Can you work these out from the model? Positions are in its coordinate system, mm. Face numbers are marked on the shaded views. A direction names the side the tool comes from. Round coordinates to 2 decimals unless told otherwise and drop trailing zeros. Write each loop counter-clockwise with the first axis right and the second up, starting at its lowest first coordinate (ties: lowest second). Pieces come first, ordered by that corner, then holes. Notation, with made-up numbers: (3, 6) -> (52, 6) arc R15 cw to (52, 19) -> close; hole circle Ø9 at (68, 46.25). An arc over 180 degrees is marked (long way). Use CSV: the item, a comma, the result in double quotes.
```python
from build123d import *

# Parameters (mm, degrees)
SKETCH1_R                            = 20.334999999999997
SKETCH1_R_2                          = 13.334999999999999
BOSS_EXTRUDE1_DEPTH                  = 12
BOSS_EXTRUDE2_DEPTH                  = 10
BOSS_EXTRUDE2_DIRECTION_2_REACH      = 49.027
BOSS_EXTRUDE2_DIRECTION_2_END_RADIUS = 13.334999999999999
CUT_EXTRUDE1_REACH                   = 62.473
CUT_EXTRUDE1_END_RADIUS              = 20.334999999999997
BOSS_EXTRUDE3_DEPTH                  = 11


with BuildPart() as part:
    # Sketch1 → Boss-Extrude1 (new body)
    with BuildSketch(Plane(origin=(0, 0, 0), x_dir=(1, 0, 0), z_dir=(0, 1, 0))):
        with Locations(Location((0, 0, 0), (0, 0, 270))):
            Circle(SKETCH1_R)
        with Locations(Location((0, 0, 0), (0, 0, 270))):
            Circle(SKETCH1_R_2, mode=Mode.SUBTRACT)
    extrude(amount=BOSS_EXTRUDE1_DEPTH)

    # Sketch2 → Boss-Extrude2 (add)
    with BuildSketch(Plane.XY.offset(20.334999999999997)):
        Polygon((-8, 26.000000000000004), (-7.9999999999999964, 0), (8.000000000000004, 0), (8, 26.000000000000004), align=None)
        Polygon((-5.000000000000001, 23.000000000000004), (5, 23.000000000000004), (4.999999999999998, 3), (-4.999999999999998, 3), align=None, mode=Mode.SUBTRACT)
    extrude(amount=BOSS_EXTRUDE2_DEPTH)

    # Boss-Extrude2 direction 2: up to this cylinder (the profile starts outside it)
    boss_extrude2_direction_2_end = Plane(origin=(0, 13, 0), z_dir=(0, -1, 0)) * Cylinder(BOSS_EXTRUDE2_DIRECTION_2_END_RADIUS, 125.724, mode=Mode.PRIVATE)
    # Sketch2 → Boss-Extrude2 direction 2 (add, up to the surface)
    with BuildSketch(Plane.XY.offset(20.334999999999997), mode=Mode.PRIVATE) as boss_extrude2_direction_2_sk1:
        Polygon((-8, 26.000000000000004), (-7.9999999999999964, 0), (8.000000000000004, 0), (8, 26.000000000000004), align=None)
        Polygon((-5.000000000000001, 23.000000000000004), (5, 23.000000000000004), (4.999999999999998, 3), (-4.999999999999998, 3), align=None, mode=Mode.SUBTRACT)
    boss_extrude2_direction_2_tool1 = extrude(boss_extrude2_direction_2_sk1.sketch, amount=-BOSS_EXTRUDE2_DIRECTION_2_REACH, mode=Mode.PRIVATE) - boss_extrude2_direction_2_end
    add(boss_extrude2_direction_2_tool1.solids().sort_by_distance((-7.694713, 13, 20.335))[0])

    # Cut-Extrude1: up to this cylinder (the profile starts outside it)
    cut_extrude1_end = Plane(origin=(0, 24.5, 0), z_dir=(0, -1, 0)) * Cylinder(CUT_EXTRUDE1_END_RADIUS, 166.61599999999999, mode=Mode.PRIVATE)
    # Sketch3 → Cut-Extrude1 (cut, up to the surface)
    with BuildSketch(Plane.XY.offset(30.335), mode=Mode.PRIVATE) as cut_extrude1_sk1:
        Polygon((-5.000000000000002, 26.000000000000004), (4.999999999999997, 26.000000000000004), (4.999999999999997, 23.000000000000004), (-5.000000000000001, 23.000000000000004), align=None)
    cut_extrude1_tool1 = extrude(cut_extrude1_sk1.sketch, amount=-CUT_EXTRUDE1_REACH, mode=Mode.PRIVATE) - cut_extrude1_end
    add(cut_extrude1_tool1.solids().sort_by_distance((0, 24.5, 30.335))[0], mode=Mode.SUBTRACT)

    # Sketch4 → Boss-Extrude3 (add)
    with BuildSketch(Plane(origin=(0, 12, 0), x_dir=(1, 0, 0), z_dir=(0, 1, 0))):
        with BuildLine():
            Line((4.999999999999998, -19.710713457406865), (4.9999999999999964, -12.362128659741414))
            ThreePointArc((4.9999999999999964, -12.362128659741414), (-2.14e-15, -13.335), (-5.000000000000001, -12.362128659741412))
            Line((-5.000000000000001, -12.362128659741412), (-5.000000000000008, -19.710713457406865))
            ThreePointArc((-5.000000000000008, -19.710713457406865), (-7.79e-15, -20.335000000000004), (4.999999999999998, -19.710713457406865))
        make_face()
    extrude(amount=BOSS_EXTRUDE3_DEPTH)


solid = part.part
```
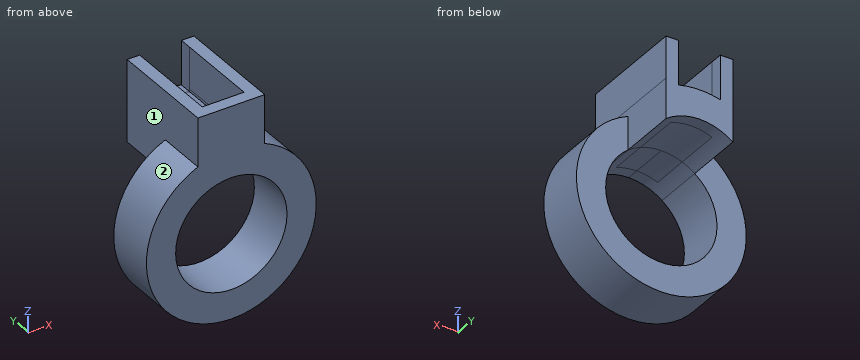
Q1. Suppose I cut it at A-A (z = 0). Write out the boundary of the cut face in (x, y) (3 decimals), and give its area (3 significant figures).
Resolved:
outline,"(-20.335, 0) -> (-13.335, 0) -> (-13.335, 12) -> (-20.335, 12) -> close; (13.335, 0) -> (20.335, 0) -> (20.335, 12) -> (13.335, 12) -> close"
area,"168 mm^2"
Q2. Suppose I cut it at C-C (y = 13). Write out the boundary of the cut face in (x, z) (3 decimals), and give its area (3 significant figures).
Resolved:
outline,"(-8, 10.669) arc R13.335 cw to (8, 10.669) -> (8, 30.335) -> (5, 30.335) -> (5, 19.711) arc R20.335 ccw to (-5, 19.711) -> (-5, 30.335) -> (-8, 30.335) -> close"
area,"184 mm^2"
Q3. Please list where these lines run through material, in increasing order: probe 1 along Z at (x, y) = (0, 4) (3 decimals); probe 2 along Y at (x, z) = (13, -5.5).
Resolved:
probe 1,"z = -20.335 to -13.335, 13.335 to 20.335"
probe 2,"y = 0 to 12"
Q4. Will these pins go through, and if not, where does the flat tip stop? P1, Ø6, axis at x = -11.5, y = 4.5, coming from the -Z side; P2, Ø1.5, axis at y = 24, z = 27.5, coming from the +X side; P3, Ø5, axis at y = 9.5, z = 24.5, coming from the -X side; P4, Ø6, axis at y = 17, z = 5.5, coming from the +X side.
Resolved:
P1,"stops at z = -18.47"
P2,"stops at x = 8"
P3,"stops at x = -8"
P4,"passes through"
Q5. On a 3-axis mill with a long thin cutter (end or side, diameter ignored), from which of +Z, -Z, +X, -X, +Y, -Y can I reach the whole of each face in a straight line? I mean the marked faces 1 and 2. Say none if no direction works.
Resolved:
face 1,"+Z, -X, +Y"
face 2,"+Y, -Y"
Q6. Suppose I cut it at D-D (y = 9). Write out the boundary of the cut face in (x, z) (3 decimals).
Resolved:
outline,"(-8, 18.695) arc R20.335 ccw (long way) to (8, 18.695) -> (8, 30.335) -> (5, 30.335) -> (5, 19.711) arc R20.335 ccw to (-5, 19.711) -> (-5, 30.335) -> (-8, 30.335) -> close; hole circle Ø26.67 at (0, 0)"
Q7. Suppose I cut it at B-B (x = -11). Write out the boundary of the cut face in (y, z).
Resolved:
outline,"(0, -17.1) -> (12, -17.1) -> (12, -7.54) -> (0, -7.54) -> close; (0, 7.54) -> (12, 7.54) -> (12, 17.1) -> (0, 17.1) -> close"
